Could you check a few things on this model? Use its own coordinates, in mm. Coordinates: 2 decimals unless noted, no trailing zeros. Write each loop counter-clockwise with the first axis right and the second up, starting at its lowest first coordinate (ties: lowest second). Pieces come first, ordered by that corner, then holes. Notation, with made-up numbers: (25.5, -21.5) - (54.5, -21.5) arc R23 cw to (54.5, 10.5) - close; hole circle Ø8 at (77, 16.25). An arc over 180 degrees is marked (long way). Answer as a JSON object with one key per item and string values. Group by question number.
1) Will this pin go through, and if not, where does the flat tip stop? pin 1 Ø3 at (x, y) = (24, -12) entering from -Z.
2) If we section it at B-B (x = 14): Write out the boundary of the cut face in (y, z).
3) Please list where these lines run through material, in increasing order: line 1 along Y through (x, z) = (-14, 4.5); line 2 along Y through (x, z) = (24, 2.25); line 3 along X through (y, z) = (13, 7.5).
4) We'd pull the mould along Y, two halves only. Please class faces 1 (the cylindrical face through (23.46, -14.44, 5.07)), 2 (the flat face through (0, 20, 5)), 3 (the flat face through (0, -20, 5)): released by +Y, released by -Y, zero draft, split by the parting line, or undercut.
5) If we section it at A-A (y = 0): Write out the boundary of the cut face in (x, z), plus the area to 3 significant figures.
6) If we section it at D-D (z = 4.5): State how many separate pieces and enclosed holes the cut face has, plus the area to 3 significant figures.
7) If we section it at C-C (y = 10.5): Write out the boundary of the cut face in (x, z).
```python
from build123d import *

# Parameters (mm, degrees)
SKETCH_1_R          = 9
EXTRUDE_1_DEPTH     = 10
SKETCH_3_R          = 2.5
CUT_EXTRUDE_1_DEPTH = 11


with BuildPart() as part:
    # ｽｹｯﾁ1 → ﾎﾞｽ - 押し出し1 (new body)
    with BuildSketch(Plane.XY):
        with BuildLine():
            Line((-25, 20), (25, 20))
            ThreePointArc((25, 20), (28.535533906, 18.535533906), (30, 15))
            Line((30, 15), (30, -15))
            ThreePointArc((30, -15), (28.535533906, -18.535533906), (25, -20))
            Line((25, -20), (-25, -20))
            ThreePointArc((-25, -20), (-28.535533906, -18.535533906), (-30, -15))
            Line((-30, -15), (-30, 15))
            ThreePointArc((-30, 15), (-28.535533906, 18.535533906), (-25, 20))
        make_face()
        Circle(SKETCH_1_R, mode=Mode.SUBTRACT)
    extrude(amount=EXTRUDE_1_DEPTH)

    # ｽｹｯﾁ3 → ｶｯﾄ - 押し出し1 (cut, through all)
    with BuildSketch(Plane.XY.offset(10)):
        with Locations((14, 6)):
            Circle(SKETCH_3_R)
        with Locations((24, 0)):
            Circle(SKETCH_3_R)
        with Locations((24, 12)):
            Circle(SKETCH_3_R)
        with Locations((24, -12)):
            Circle(SKETCH_3_R)
        with Locations((14, -6)):
            Circle(SKETCH_3_R)
    cut_extrude_1 = extrude(amount=-CUT_EXTRUDE_1_DEPTH, mode=Mode.SUBTRACT)

    # ﾐﾗｰ1: ｶｯﾄ - 押し出し1 across plane
    add(cut_extrude_1.mirror(Plane(origin=(0, 0, 0), x_dir=(0, 0, 1), z_dir=(1, 0, 0))), mode=Mode.SUBTRACT)


solid = part.part
```
Here are the results:
{
 "1": {"pin 1": "passes through"},
 "2": {"outline": "(-20, 0) - (-8.5, 0) - (-8.5, 10) - (-20, 10) - close; (-3.5, 0) - (3.5, 0) - (3.5, 10) - (-3.5, 10) - close; (8.5, 0) - (20, 0) - (20, 10) - (8.5, 10) - close"},
 "3": {"line 1": "y = -20 to -8.5, -3.5 to 3.5, 8.5 to 20", "line 2": "y = -20 to -14.5, -9.5 to -2.5, 2.5 to 9.5, 14.5 to 20", "line 3": "x = -30 to -26.29, -21.71 to 21.71, 26.29 to 30"},
 "4": {"face 1": "undercut", "face 2": "released by +Y", "face 3": "released by -Y"},
 "5": {"outline": "(-30, 0) - (-26.5, 0) - (-26.5, 10) - (-30, 10) - close; (-21.5, 0) - (-9, 0) - (-9, 10) - (-21.5, 10) - close; (9, 0) - (21.5, 0) - (21.5, 10) - (9, 10) - close; (26.5, 0) - (30, 0) - (30, 10) - (26.5, 10) - close", "area": "320 mm²"},
 "6": {"separate pieces": "1", "enclosed holes": "11", "area": "1,930 mm²"},
 "7": {"outline": "(-30, 0) - (-26, 0) - (-26, 10) - (-30, 10) - close; (-22, 0) - (22, 0) - (22, 10) - (-22, 10) - close; (26, 0) - (30, 0) - (30, 10) - (26, 10) - close"}
}
